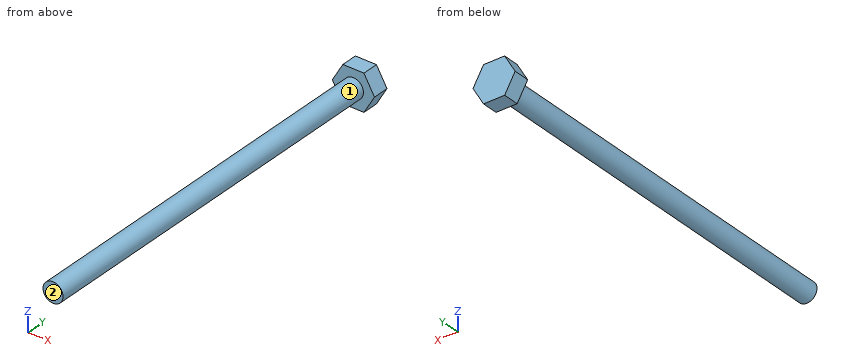
Autodesk Inventor part; units mm, degrees
ref_plane "YZ Plane" through (0, 0, 0) normal (1, 0, 0) x (0, 1, 0)
ref_plane "XZ Plane" through (0, 0, 0) normal (0, 1, 0) x (-1, 0, 0)
ref_plane "XY Plane" through (0, 0, 0) normal (0, 0, 1) x (1, 0, 0)
sketch "Sketch1" plane through (0, 0, 0) normal (0, 1, 0) x (-1, 0, 0)
  circle A0 centre (0, 0) radius 1.9844
  dimension "d0" = 3.9688
extrude "Extrusion1" add sketch "Sketch1" along normal blind 76.2
sketch "Sketch2" plane through (0, 76.2, 0) normal (0, 1, 0) x (1, 0, 0)
  line L0 (-4.1682, 0) -> (-2.0841, 3.6098)
  line L1 (-2.0841, 3.6098) -> (2.0841, 3.6098)
  line L2 (2.0841, 3.6098) -> (4.1682, 0)
  line L3 (4.1682, 0) -> (2.0841, -3.6098)
  line L4 (2.0841, -3.6098) -> (-2.0841, -3.6098)
  line L5 (-2.0841, -3.6098) -> (-4.1682, 0)
  point P0 (0, 0)
  point P1 (0, 0)
extrude "Extrusion2" add sketch "Sketch2" along normal blind 3.175
properties part number "Bag motor bolt"
The listing builds one solid part. Answer for the finished solid, in the listing's coordinates (mm). Face numbers are marked on the shaded views. A direction names the side the tool comes from. Round coordinates to 2 decimals unless told otherwise and drop trailing zeros. Loops run counter-clockwise (first coordinate to the right, second up) from the corner with the lowest first, then second, coordinate; pieces in that order, holes last.
Q1. Which of the six approach directions +Z, -Z, +X, -X, +Y, -Y give full straight-line access (tool end or side, diameter ignored) to the marked faces 1 and 2?
Q2. Section C-C, the plane z = 2.75 is taken. Determine the outline of the cut face in (x, y) (1 decimal).
Q3. Find the intervals of material crossed by line 1 (Y direction, x = -2, z = 0.5) (3 decimals); line 2 (Z direction, x = -1.75, y = 10); line 3 (X direction, y = 63.5, z = -0.75), in increasing order.
Q4. Given pin 1 Ø4 at (x, z) = (2, 2) entering from -Y; pin 2 Ø1 at (y, z) = (65, 2) entering from -X; pin 3 Ø3 at (y, z) = (57, 0.5) entering from -X, each flat-ended and moving along its own axis, determine where each tip first touches the part or whether it passes through.
Q5. Section A-A, the plane x = 0 is taken. Determine the outline of the cut face in (y, z) (3 decimals).
Q6. Section B-B, the plane y = 59 is taken. Determine the outline of the cut face in (x, z).
Q7. Section D-D, the plane x = 3.5 is taken. Determine the outline of the cut face in (y, z) (3 decimals).
Completed:
1. face 1: -Y
1. face 2: +Z, -Z, +X, -X, -Y
2. outline: (-2.6, 76.2) - (2.6, 76.2) - (2.6, 79.4) - (-2.6, 79.4) - close
3. line 1: y = 76.2 to 79.375
3. line 2: z = -0.94 to 0.94
3. line 3: x = -1.84 to 1.84
4. pin 1: stops at y = 0
4. pin 2: stops at x = -1.3
4. pin 3: stops at x = -1.98
5. outline: (0, -1.984) - (76.2, -1.984) - (76.2, -3.61) - (79.375, -3.61) - (79.375, 3.61) - (76.2, 3.61) - (76.2, 1.984) - (0, 1.984) - close
6. outline: circle Ø3.97 at (0, 0)
7. outline: (76.2, -1.157) - (79.375, -1.157) - (79.375, 1.157) - (76.2, 1.157) - close
